```python
from build123d import *

# Parameters (mm, degrees)
CROQUIS1_W              = 84
CROQUIS1_H              = 70
SALIENTE_EXTRUIR1_DEPTH = 3
CROQUIS2_W              = 6
CROQUIS2_H              = 10
CORTAR_EXTRUIR1_DEPTH   = 3
CROQUIS3_W              = 20
CROQUIS3_H              = 3
CROQUIS3_W_2            = 3
CROQUIS3_H_2            = 20
CORTAR_EXTRUIR2_DEPTH   = 3
CORTAR_EXTRUIR3_DEPTH   = 146


with BuildPart() as part:
    # Croquis1 → Saliente-Extruir1 (new body)
    with BuildSketch(Plane(origin=(0, 0, 0), x_dir=(1, 0, 0), z_dir=(0, 1, 0))):
        Polygon((72.5, 73.5), (-72.5, 73.5), (-72.5, -3.5), (-42, -3.5), (42, -3.5), (72.5, -3.5), align=None)
        with Locations((0, -38.5)):
            Rectangle(CROQUIS1_W, CROQUIS1_H)
    extrude(amount=SALIENTE_EXTRUIR1_DEPTH)

    # Croquis2 → Cortar-Extruir1 (cut)
    with BuildSketch(Plane(origin=(0, 3, 0), x_dir=(1, 0, 0), z_dir=(0, 1, 0))):
        with Locations((-34.09, -62.5)):
            Rectangle(CROQUIS2_W, CROQUIS2_H)
        with Locations((34.09, -62.5)):
            Rectangle(CROQUIS2_W, CROQUIS2_H)
        with Locations((-58.11, 50.77)):
            Rectangle(CROQUIS2_W, CROQUIS2_H)
        with Locations((58.11, 50.77)):
            Rectangle(CROQUIS2_W, CROQUIS2_H)
    extrude(amount=-CORTAR_EXTRUIR1_DEPTH, mode=Mode.SUBTRACT)

    # Croquis3 → Cortar-Extruir2 (cut)
    with BuildSketch(Plane(origin=(0, 3, 0), x_dir=(1, 0, 0), z_dir=(0, 1, 0))):
        with Locations((0, -72)):
            Rectangle(CROQUIS3_W, CROQUIS3_H)
        with Locations((71, 35)):
            Rectangle(CROQUIS3_W_2, CROQUIS3_H_2)
        with Locations((-71, 35)):
            Rectangle(CROQUIS3_W_2, CROQUIS3_H_2)
        with Locations((57.25, -2)):
            Rectangle(CROQUIS3_W, CROQUIS3_H)
        with Locations((-57.25, -2)):
            Rectangle(CROQUIS3_W, CROQUIS3_H)
    extrude(amount=-CORTAR_EXTRUIR2_DEPTH, mode=Mode.SUBTRACT)

    # Croquis5 → Cortar-Extruir3 (cut, through all)
    with BuildSketch(Plane(origin=(72.5, 0, 0), x_dir=(0, 0, -1), z_dir=(1, 0, 0))):
        Polygon((73.5, 0), (70.5, 3), (73.5, 3), align=None)
    extrude(amount=-CORTAR_EXTRUIR3_DEPTH, mode=Mode.SUBTRACT)


solid = part.part
```
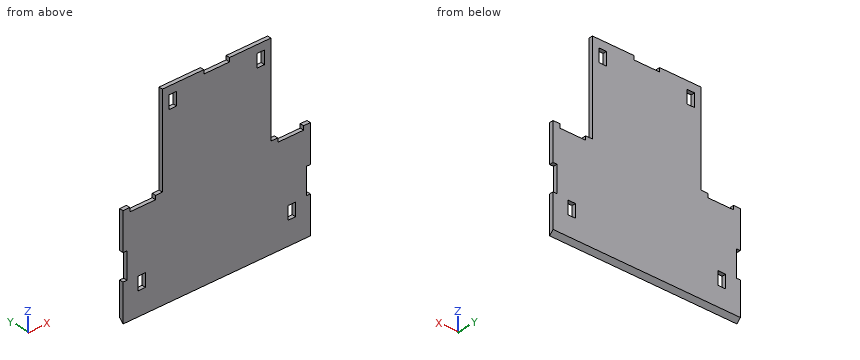
Geometry check sheet. Reference: the model listing, model coordinates, mm. Round coordinates to 2 decimals unless told otherwise and drop trailing zeros. Order: outer loops, then holes, each group sorted by start corner. A loop starts at its lowest first (then second) coordinate and runs counter-clockwise, first axis right, second up. Notation, with made-up numbers: (18.5, 39) -> (29.5, 39) arc R14 ccw to (29.5, 56) -> close; hole circle Ø5 at (36, 23). An arc over 180 degrees is marked (long way). Return JSON: item names as keys, results as strings. Group by question number.
Q1. Section check C-C, the plane z = 18. Record the boundary of the cut face in (x, y), plus the area to 3 significant figures.
Q2. Section check D-D, the plane x = -4. Record the boundary of the cut face in (y, z).
Q3. Section check A-A, the plane z = -51.5. Record the boundary of the cut face in (x, y).
Q4. Gauge pin test, flat ends, axial feed: pin 1 (0.9 mm diameter, centred on x = -4, y = 2, fed in from +Z); pin 2 (1 mm diameter, centred on x = -52.5, y = 2.5, fed in from -Z); pin 3 (1.5 mm diameter, centred on y = 1.5, z = 22.5, fed in from -X). Record the tip position at first contact, or that the pin passes through.
Q5. Material ranges on probe 1 along Z at (x, y) = (27.5, 1); probe 2 along X at (y, z) = (2.15, 4); probe 3 along X at (y, z) = (1.8, -42), recorded low to high. Write a range as from..to.
Q6. Section check B-B, the plane y = 0.65. Count the separate pieces of the cut face and the enclosed holes in it, plus the area to 3 significant figures.
Numbers:
{
 "1": {"outline": "(-42, 0) -> (42, 0) -> (42, 3) -> (-42, 3) -> close", "area": "252 mm^2"},
 "2": {"outline": "(0, -73.5) -> (3, -70.5) -> (3, 70.5) -> (0, 70.5) -> close"},
 "3": {"outline": "(-72.5, 0) -> (-61.11, 0) -> (-61.11, 3) -> (-72.5, 3) -> close; (-55.11, 0) -> (55.11, 0) -> (55.11, 3) -> (-55.11, 3) -> close; (61.11, 0) -> (72.5, 0) -> (72.5, 3) -> (61.11, 3) -> close"},
 "4": {"pin 1": "z = 70.5", "pin 2": "z = -71.5", "pin 3": "x = -42"},
 "5": {"probe 1": "-72.5..73.5", "probe 2": "-42..42", "probe 3": "-69.5..69.5"},
 "6": {"separate pieces": "1", "enclosed holes": "4", "area": "16,400 mm^2"}
}
